from build123d import *

# Parameters (mm, degrees)
SKETCH1_R           = 3.15
BOSS_EXTRUDE1_DEPTH = 5.9
FILLET1_R           = 3


with BuildPart() as part:
    # Sketch1 → Boss-Extrude1 (new body)
    with BuildSketch(Plane.XY):
        with BuildLine():
            Line((25.7175, -8), (-25.7175, -8))
            ThreePointArc((-25.7175, -8), (-33.7175, 0), (-25.7175, 8))
            Line((-25.7175, 8), (-9.155600281, 8))
            ThreePointArc((-9.155600281, 8), (-4.155600281, 3), (0.844399719, 8))
            Line((0.844399719, 8), (25.7175, 8))
            ThreePointArc((25.7175, 8), (33.7175, 0), (25.7175, -8))
        make_face()
        with Locations((25.7175, 0)):
            Circle(SKETCH1_R, mode=Mode.SUBTRACT)
        with Locations((-25.7175, 0)):
            Circle(SKETCH1_R, mode=Mode.SUBTRACT)
    extrude(amount=BOSS_EXTRUDE1_DEPTH)

    # Fillet1
    fillet1_edges = [part.edges().sort_by_distance(p)[0] for p in [
        (-9.155600281, 8, 2.95),
        (0.844399719, 8, 2.95),
    ]]
    fillet(fillet1_edges, radius=FILLET1_R)


solid = part.part
CAD build for the part. Positions are in the model's coordinates, mm. A direction names the side the tool comes from. Give positions to 0.01 mm unless a question says otherwise; leave off trailing zeros. Loops run counter-clockwise (first coordinate to the right, second up) from the corner with the lowest first, then second, coordinate; pieces in that order, holes last. Notation, with made-up numbers: M 52.25,24 L 101.25,24 A32 cw 101.25,58 Z; hole C 23,22 d5. An arc over 180 degrees is marked long. Write each question's results on one line, items separated by ' | '.
Q1. Band-saw the part on C-C on y = 4. Write the cut outline in (x, z), and give its area (3 significant figures).
Geometry check:
outline: M -32.65,0 L -7.16,0 L -7.16,5.9 L -32.65,5.9 Z; M -1.16,0 L 32.65,0 L 32.65,5.9 L -1.16,5.9 Z | area: 350 mm²
Q2. Which spindle directions (+Z, -Z, +X, -X, +Y, -Y) get a long thin tool onto all of the face, cutting with end or side? Do faces 1 (the face through (33.716, 0.176, 2.909)), 2 (the face through (-9.915, 7.501, 2.991)). Say none if no direction does.
Geometry check:
face 1: +Z, -Z, +X | face 2: +Z, -Z, +Y
Q3. Band-saw the part on D-D on x = -0.5. Write the cut outline in (y, z).
Geometry check:
outline: M -8,0 L 4.59,0 L 4.59,5.9 L -8,5.9 Z
Q4. Mould opens along Y. For faces 3 (the face through (-19, 8, 3)), 4 (the face through (22.57, 0.14, 2.91)), 5 (the face through (-33.716, -0.176, 2.909)), 6 (the face through (-28.864, 0.138, 2.909)) say: pulls with the +Y half, pulls with the -Y half, needs draft (parallel to the pull), parting line crosses it, or undercut.
Geometry check:
face 3: pulls with the +Y half | face 4: undercut | face 5: parting line crosses it | face 6: undercut
Q5. Flat gauge pins, fed straight in: P1, Ø3, axis at y = 3, z = 5, coming from the -X side; P2, Ø8, axis at x = 25.72, y = 0, coming from the -Z side; P3, Ø1.5, axis at y = 1.5, z = 4.5, coming from the -X side; P4, Ø1.5, axis at y = 4.5, z = 4.5, coming from the +X side. Where does each tip first touch, or does it go through?
Geometry check:
P1: stops at x = -33.58 | P2: stops at z = 0 | P3: stops at x = -33.68 | P4: stops at x = 32.78
Q6. Band-saw the part on B-B on y = 0. Write the cut outline in (x, z).
Geometry check:
outline: M -33.72,0 L -28.87,0 L -28.87,5.9 L -33.72,5.9 Z; M -22.57,0 L 22.57,0 L 22.57,5.9 L -22.57,5.9 Z; M 28.87,0 L 33.72,0 L 33.72,5.9 L 28.87,5.9 Z
Q7. Probe probe 1 along X at (y, z) = (-0.25, 5.6); probe 2 along X at (y, z) = (-1, 1.5); probe 3 along Y at (x, z) = (-26, 5.45). List the from-to ranges inside material, lowest first.
Geometry check:
probe 1: x = -33.71 to -28.86, -22.58 to 22.58, 28.86 to 33.71 | probe 2: x = -33.65 to -28.7, -22.73 to 22.73, 28.7 to 33.65 | probe 3: y = -8 to -3.14, 3.14 to 8
Q8. Band-saw the part on A-A on z = 4.55. Give the number of separate pieces and of enclosed holes in the cut face, and give its area (3 significant figures).
Geometry check:
separate pieces: 1 | enclosed holes: 2 | area: 920 mm²
